Input: part model. Units: mm. Frame: model coordinates. A direction names the side the tool comes from. Give positions to 0.01 mm unless a question says otherwise; leave off trailing zeros. Loops run counter-clockwise (first coordinate to the right, second up) from the corner with the lowest first, then second, coordinate; pieces in that order, holes last. Notation, with made-up numbers: (72, 12) - (111, 12) arc R21 cw to (111, 36) - close; hole circle Ø7 at (56, -5). An arc over 180 degrees is marked (long way). Answer as a JSON object with one key per item and string values.
from build123d import *

# Parameters (mm, degrees)
SKETCH1_W           = 25.4
SKETCH1_H           = 25.4
SKETCH1_W_2         = 22.225
SKETCH1_H_2         = 22.225
BOSS_EXTRUDE1_DEPTH = 228.6
SKETCH3_R           = 2.54
CUT_EXTRUDE2_DEPTH  = 232.40501291
SKETCH4_R           = 2.54
CUT_EXTRUDE3_DEPTH  = 232.40501291


with BuildPart() as part:
    # Sketch1 → Boss-Extrude1 (new body)
    with BuildSketch(Plane.XY):
        with Locations((12.7, 12.7)):
            Rectangle(SKETCH1_W, SKETCH1_H)
        with Locations((12.7, 12.7)):
            Rectangle(SKETCH1_W_2, SKETCH1_H_2, mode=Mode.SUBTRACT)
    extrude(amount=BOSS_EXTRUDE1_DEPTH)

    # Sketch3 → Cut-Extrude2 (cut, through all)
    with BuildSketch(Plane(origin=(0, 25.4, 0), x_dir=(1, 0, 0), z_dir=(0, 1, 0))):
        with Locations(Location((15.875, -215.9, 0), (0, 0, 270))):
            Circle(SKETCH3_R)
        with Locations(Location((15.875, -12.7, 0), (0, 0, 270))):
            Circle(SKETCH3_R)
    extrude(amount=-CUT_EXTRUDE2_DEPTH, mode=Mode.SUBTRACT)

    # Sketch4 → Cut-Extrude3 (cut, through all)
    with BuildSketch(Plane(origin=(25.4, 0, 0), x_dir=(0, 0, -1), z_dir=(1, 0, 0))):
        with Locations((-215.9, 12.7)):
            Circle(SKETCH4_R)
        with Locations((-190.5, 12.7)):
            Circle(SKETCH4_R)
        with Locations((-165.1, 12.7)):
            Circle(SKETCH4_R)
        with Locations((-139.7, 12.7)):
            Circle(SKETCH4_R)
        with Locations((-114.3, 12.7)):
            Circle(SKETCH4_R)
        with Locations((-88.9, 12.7)):
            Circle(SKETCH4_R)
        with Locations((-63.5, 12.7)):
            Circle(SKETCH4_R)
        with Locations((-38.1, 12.7)):
            Circle(SKETCH4_R)
        with Locations((-12.7, 12.7)):
            Circle(SKETCH4_R)
    extrude(amount=-CUT_EXTRUDE3_DEPTH, mode=Mode.SUBTRACT)


solid = part.part
Item 1: Cut plane B-B (x = 9). Return loops of the section in (y, z), then the cut area to 3 significant figures.
Geometry check:
{"outline": "(0, 0) - (1.59, 0) - (1.59, 228.6) - (0, 228.6) - close; (23.81, 0) - (25.4, 0) - (25.4, 228.6) - (23.81, 228.6) - close", "area": "726 mm2"}
Item 2: Material intervals for line 1 (Y direction, x = 9.25, z = 127); line 2 (X direction, y = 25.05, z = 12.7) (3 decimals), sorted ascending. Write a range as [from, to].
Geometry check:
{"line 1": "y = [0, 1.59], [23.81, 25.4]", "line 2": "x = [0, 13.335], [18.415, 25.4]"}
Item 3: Contact query for a flat-ended pin moving along its axis: P1, Ø4, axis at y = 12.7, z = 215.9, coming from the +X side. Output: stop coordinate, or through.
Geometry check:
{"P1": "passes through"}
Item 4: Cut plane C-C (z = 63.5). Return loops of the section in (x, y), then the cut area to 3 significant figures.
Geometry check:
{"outline": "(0, 0) - (25.4, 0) - (25.4, 10.16) - (23.81, 10.16) - (23.81, 1.59) - (1.59, 1.59) - (1.59, 10.16) - (0, 10.16) - close; (0, 15.24) - (1.59, 15.24) - (1.59, 23.81) - (23.81, 23.81) - (23.81, 15.24) - (25.4, 15.24) - (25.4, 25.4) - (0, 25.4) - close", "area": "135 mm2"}
Item 5: Mould query, pull axis Y, two halves, no side actions, for faces 1 (the face through (25.4, 15.3, 112.7)), 2 (the face through (23.812, 15, 112.7)), 3 (the face through (13, 0, 113)). Classes: released by +Y, released by -Y, zero draft, split by the parting line, or undercut.
Geometry check:
{"face 1": "zero draft", "face 2": "undercut", "face 3": "released by -Y"}
Item 6: Access query for faces 4 (the face through (0, 15.3, 112.7)), 5 (the face through (13, 23.812, 113)). Directions: +Z, -Z, +X, -X, +Y, -Y. A direction counts if a zero-diameter tool reaches every point of the face in a straight line with its end or side. Return the directions, or none.
Geometry check:
{"face 4": "+Z, -Z, -X, +Y, -Y", "face 5": "+Z, -Z"}
Item 7: Cut plane A-A (z = 12.7). Return loops of the section in (x, y) (1 decimal), then the cut area to 3 significant figures.
Geometry check:
{"outline": "(0, 0) - (13.3, 0) - (13.3, 1.6) - (1.6, 1.6) - (1.6, 10.2) - (0, 10.2) - close; (0, 15.2) - (1.6, 15.2) - (1.6, 23.8) - (13.3, 23.8) - (13.3, 25.4) - (0, 25.4) - close; (18.4, 0) - (25.4, 0) - (25.4, 10.2) - (23.8, 10.2) - (23.8, 1.6) - (18.4, 1.6) - close; (18.4, 23.8) - (23.8, 23.8) - (23.8, 15.2) - (25.4, 15.2) - (25.4, 25.4) - (18.4, 25.4) - close", "area": "119 mm2"}
